Work out the finished part from the listing and answer in its coordinate system (mm). Coordinates: 2 decimals unless noted, no trailing zeros. Loops run counter-clockwise (first coordinate to the right, second up) from the corner with the lowest first, then second, coordinate; pieces in that order, holes last. Notation, with made-up numbers: (78.25, 8) - (111.25, 8) arc R30 ccw to (111.25, 31) - close; hole circle Ø11 at (28.5, 82). An arc over 180 degrees is marked (long way). Write each question's results on one line, items separated by ' | '. Start each with the question number.
Item 1: Each of these flat-tipped pins is pushed along its axis until it touches: pin 1 Ø2.5 at (x, z) = (147, -154.43) entering from +Y; pin 2 Ø1.5 at (x, y) = (113, 3) entering from +Z; pin 3 Ø2 at (x, y) = (-2.5, 2) entering from -Z. Where does it stop, or does it pass through?
Item 2: Consider probe 1 along Z at (x, y) = (48, 3.1); probe 2 along Z at (x, y) = (111.5, 1.85); probe 3 along X at (y, z) = (2.05, -26). Determine where each line is inside the solid, lowest interval first. Write a range as [from, to].
Item 3: Section A-A, the plane x = 98 is taken. Write down the section's boundary in (y, z).
Item 4: Section B-B, the plane z = -135 is taken. Write down the section's boundary in (x, y), plus the area to 3 significant figures.
Item 5: Section C-C, the plane x = 13 is taken. Write down the section's boundary in (y, z).
Item 6: Section D-D, the plane y = 2.95 is taken. Count the separate pieces of the cut face and the enclosed holes in it, plus the area to 3 significant figures.
from build123d import *

# Parameters (mm, degrees)
SKETCH1_W                       = 210
SKETCH1_H                       = 200
BOSS_EXTRUDE1_DEPTH             = 4
SKETCH2_W                       = 40
SKETCH2_H                       = 75
CUT_EXTRUDE1_DEPTH              = 291.027584895
SKETCH5_W                       = 20
SKETCH5_H                       = 4
BOSS_EXTRUDE2_DEPTH             = 4
SKETCH6_W                       = 20
SKETCH6_H                       = 4
BOSS_EXTRUDE3_DEPTH             = 4
F_3_0MM_DOWEL_HOLE1_D           = 3
F_3_0MM_DOWEL_HOLE1_CSINK_D     = 3.05
F_3_0MM_DOWEL_HOLE1_CSINK_ANGLE = 90
SKETCH10_W                      = 45
SKETCH10_H                      = 11.5
CUT_EXTRUDE2_DEPTH              = 293.936853264
F_3_0MM_DOWEL_HOLE2_D           = 3
F_3_0MM_DOWEL_HOLE2_CSINK_D     = 3.05
F_3_0MM_DOWEL_HOLE2_CSINK_ANGLE = 90


with BuildPart() as part:
    # Sketch1 → Boss-Extrude1 (new body)
    with BuildSketch(Plane(origin=(0, 0, 0), x_dir=(1, 0, 0), z_dir=(0, 1, 0))):
        with Locations((105, 100)):
            Rectangle(SKETCH1_W, SKETCH1_H)
    extrude(amount=BOSS_EXTRUDE1_DEPTH)

    # Sketch2 → Cut-Extrude1 (cut, through all)
    with BuildSketch(Plane(origin=(0, 4, 0), x_dir=(1, 0, 0), z_dir=(0, 1, 0))):
        with Locations((190, 162.5)):
            Rectangle(SKETCH2_W, SKETCH2_H)
        with Locations((20, 162.5)):
            Rectangle(SKETCH2_W, SKETCH2_H)
    extrude(amount=-CUT_EXTRUDE1_DEPTH, mode=Mode.SUBTRACT)

    # Sketch5 → Boss-Extrude2 (add)
    with BuildSketch(Plane(origin=(210, 0, 0), x_dir=(0, 0, -1), z_dir=(1, 0, 0))):
        with Locations((95, 2)):
            Rectangle(SKETCH5_W, SKETCH5_H)
        with Locations((40, 2)):
            Rectangle(SKETCH5_W, SKETCH5_H)
    extrude(amount=BOSS_EXTRUDE2_DEPTH)

    # Sketch6 → Boss-Extrude3 (add)
    with BuildSketch(Plane.ZY):
        with Locations((-95, 2)):
            Rectangle(SKETCH6_W, SKETCH6_H)
        with Locations((-40, 2)):
            Rectangle(SKETCH6_W, SKETCH6_H)
    extrude(amount=BOSS_EXTRUDE3_DEPTH)

    # Ø3.0mm Dowel Hole1 (through all)
    with Locations(Plane(origin=(0, 4, 0), x_dir=(1, 0, 0), z_dir=(0, 1, 0))):
        with Locations((137.499998178, 34.210002794), (82.5, 34.22415936), (162, 170.432778178), (162, 154.432778178), (147, 154.432778178), (147, 170.432778178), (63, 170.432778178), (48, 170.432778178), (48, 154.432778178), (63, 154.432778178), (189.704460004, 108.892072525), (189.704460004, 72.150272201), (152.324959132, 72.150272201), (152.324959132, 108.892072525)):
            CounterSinkHole(F_3_0MM_DOWEL_HOLE1_D / 2, F_3_0MM_DOWEL_HOLE1_CSINK_D / 2, counter_sink_angle=F_3_0MM_DOWEL_HOLE1_CSINK_ANGLE)

    # Sketch10 → Cut-Extrude2 (cut, through all)
    with BuildSketch(Plane(origin=(0, 4, 0), x_dir=(1, 0, 0), z_dir=(0, 1, 0))):
        with Locations((110, 27.47415936)):
            Rectangle(SKETCH10_W, SKETCH10_H)
    extrude(amount=-CUT_EXTRUDE2_DEPTH, mode=Mode.SUBTRACT)

    # Ø3.0mm Dowel Hole2 (through all)
    with Locations(Plane(origin=(0, 0, 0), x_dir=(-1, 0, 0), z_dir=(0, -1, 0))):
        with Locations((-33.660254038, 6.028412794), (-173.660254038, 6.028412794)):
            CounterSinkHole(F_3_0MM_DOWEL_HOLE2_D / 2, F_3_0MM_DOWEL_HOLE2_CSINK_D / 2, counter_sink_angle=F_3_0MM_DOWEL_HOLE2_CSINK_ANGLE)


solid = part.part
Answer key:
1) pin 1: passes through | pin 2: stops at z = 0 | pin 3: stops at z = -105
2) probe 1: z = [-200, -171.93], [-168.93, -155.93], [-152.93, 0] | probe 2: z = [-200, -33.22], [-21.72, 0] | probe 3: x = [0, 87.5], [132.5, 210]
3) outline: (0, -200) - (4, -200) - (4, -33.22) - (0, -33.22) - close; (0, -21.72) - (4, -21.72) - (4, 0) - (0, 0) - close
4) outline: (40, 0) - (170, 0) - (170, 4) - (40, 4) - close | area: 520 mm^2
5) outline: (0, -125) - (4, -125) - (4, 0) - (0, 0) - close
6) separate pieces: 1 | enclosed holes: 17 | area: 35,700 mm^2
